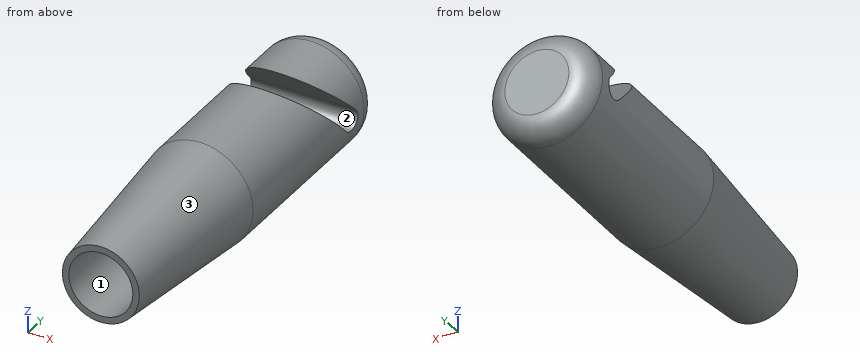
from build123d import *

# Parameters (mm, degrees)
SKETCH1_R               = 2.5
BOSS_EXTRUDE1_DEPTH     = 10
SKETCH2_R               = 2.5
BOSS_EXTRUDE2_DEPTH     = 8
BOSS_EXTRUDE2_TAPER     = 5
CUT_EXTRUDE1_START      = -8
SKETCH3_R               = 1.5
CUT_EXTRUDE1_DEPTH      = 8
FILLET1_R               = 1
CUT_EXTRUDE2_DEPTH      = 3.5000001
CUT_EXTRUDE2_DEPTH_BACK = 3.5000001


with BuildPart() as part:
    # Sketch1 → Boss-Extrude1 (new body)
    with BuildSketch(Plane(origin=(0, 0, 0), x_dir=(1, 0, 0), z_dir=(0, 1, 0))):
        Circle(SKETCH1_R)
    extrude(amount=BOSS_EXTRUDE1_DEPTH)

    # Sketch2 → Boss-Extrude2 (add)
    with BuildSketch(Plane.XZ):
        Circle(SKETCH2_R)
    extrude(amount=BOSS_EXTRUDE2_DEPTH, taper=BOSS_EXTRUDE2_TAPER)

    # Sketch3 → Cut-Extrude1 (cut)
    with BuildSketch(Plane.XZ.offset(8).offset(CUT_EXTRUDE1_START)):
        Circle(SKETCH3_R)
    extrude(amount=CUT_EXTRUDE1_DEPTH, mode=Mode.SUBTRACT)

    # Fillet1
    fillet1_edges = [part.edges().sort_by_distance(p)[0] for p in [
        (-2.5, 10, 0),
    ]]
    fillet(fillet1_edges, radius=FILLET1_R)

    # Sketch4 → Cut-Extrude2 (cut, two sides)
    with BuildSketch(Plane(origin=(0, 0, 0), x_dir=(0, 0, -1), z_dir=(1, 0, 0))) as cut_extrude2_sk:
        with BuildLine():
            Line((0.353553391, 7.646446609), (-6.418274977, 0.874618242))
            Line((-6.418274977, 0.874618242), (-6.418274977, 2.288831805))
            Line((-6.418274977, 2.288831805), (-0.353553391, 8.353553391))
            ThreePointArc((-0.353553391, 8.353553391), (0.353553391, 8.353553391), (0.353553391, 7.646446609))
        make_face()
    extrude(amount=CUT_EXTRUDE2_DEPTH, mode=Mode.SUBTRACT)
    extrude(cut_extrude2_sk.sketch, amount=-CUT_EXTRUDE2_DEPTH_BACK, mode=Mode.SUBTRACT)


solid = part.part
Source: CAD feature listing. Evaluate the final solid. Frame: model axes, mm. Face numbers are marked on the shaded views. Coordinates: 2 decimals unless noted, no trailing zeros. Order: outer loops, then holes, each group sorted by start corner. A loop starts at its lowest first (then second) coordinate and runs counter-clockwise, first axis right, second up. Notation, with made-up numbers: M 37.25,42 L 68.25,42 A14 ccw 68.25,54 Z; hole C 45.5,74.5 d2. An arc over 180 degrees is marked long. Write each question's results on one line, items separated by ' | '. Start each with the question number.
Item 1: First-contact query: pin 1 Ø1.5 at (x, z) = (0.5, 0) entering from -Y; pin 2 Ø1 at (y, z) = (8, 1) entering from -X; pin 3 Ø1 at (x, y) = (-1, 0) entering from +Z. Flat tips, straight axial feed; report the tip coordinate or a pass-through.
Item 2: Cut plane C-C (y = 1.25). Return loops of the section in (x, z), and give its area (3 significant figures).
Item 3: Draft query along X for the marked faces 1, 2 and 3. Return one class per face: pulls with the +X half, pulls with the -X half, needs draft (parallel to the pull), parting line crosses it, or undercut.
Item 4: Cut plane A-A (x = 0). Return loops of the section in (y, z), and give its area (3 significant figures).
Item 5: Cut plane D-D (y = -1). Return loops of the section in (x, z).
Item 6: Line query: probe 1 along Y at (x, z) = (-0.05, -0.9); probe 2 along Y at (x, z) = (0.8, 0.35); probe 3 along Y at (x, z) = (-1.05, 1.3). Output: solid intervals per line, ascending.
Item 7: Cut plane B-B (y = 8). Return loops of the section in (x, z), and give its area (3 significant figures).
Checked values:
1) pin 1: stops at y = 0 | pin 2: stops at x = -2.44 | pin 3: stops at z = 2.45
2) outline: C 0,0 d5 | area: 19.6 mm2
3) face 1: undercut | face 2: needs draft | face 3: parting line crosses it
4) outline: M -8,-1.8 L 0,-2.5 L 9,-2.5 A1 ccw 10,-1.5 L 10,1.5 A1 ccw 9,2.5 L 6.21,2.5 L 8.35,0.35 A0.5 cw 7.65,-0.35 L 4.79,2.5 L 0,2.5 L -8,1.8 L -8,1.5 L 0,1.5 L 0,-1.5 L -8,-1.5 Z | area: 56.0 mm2
5) outline: C 0,0 d4.83; hole C 0,0 d3
6) probe 1: y = 0 to 10 | probe 2: y = 0 to 6.94, 8.36 to 10 | probe 3: y = -8 to 5.99, 7.41 to 9.99
7) outline: M -2.45,-0.5 A2.5 ccw 2.45,-0.5 Z; M -2.4,0.71 L 2.4,0.71 A2.5 ccw Z | area: 13.7 mm2
